```python
from build123d import *

# Parameters (mm, degrees)
BOSS_EXTRUDE1_DEPTH  = 10.16
SKETCH3_R            = 1.27
CUT_EXTRUDE1_DEPTH   = 10.16
SKETCH4_W            = 8.255
SKETCH4_H            = 7.62
CUT_EXTRUDE2_DEPTH   = 10.16
FILLET2_R            = 0.508
FILLET3_R            = 1.27
SKETCH6_W            = 84.495652993
SKETCH6_H            = 50.182540269
CUT_EXTRUDE3_DEPTH   = 27.94
CUT_EXTRUDE4_DEPTH   = 27.94
CUT_EXTRUDE5_DEPTH   = 40.132
FILLET4_R            = 2.54
FILLET2_OF_MIRROR1_R = 0.508
FILLET3_OF_MIRROR1_R = 1.27
FILLET4_OF_MIRROR1_R = 2.54


with BuildPart() as part:
    # Sketch1 → Boss-Extrude1 (new body)
    with BuildSketch(Plane(origin=(0, 0, 0), x_dir=(1, 0, 0), z_dir=(0, 1, 0))):
        with BuildLine():
            Line((-58.188733064, -33.517116066), (5.311266936, -33.517116066))
            Line((5.311266936, -33.517116066), (5.311266936, 14.742883934))
            Line((5.311266936, 14.742883934), (-53.108733064, 14.742883934))
            ThreePointArc((-53.108733064, 14.742883934), (-56.700835512, 13.254986382), (-58.188733064, 9.662883934))
            Line((-58.188733064, 9.662883934), (-58.188733064, -0.370116066))
            Line((-58.188733064, -0.370116066), (-66.443733064, -0.370116066))
            Line((-66.443733064, -0.370116066), (-66.443733064, -5.450116066))
            Line((-66.443733064, -5.450116066), (-58.188733064, -5.450116066))
            Line((-58.188733064, -5.450116066), (-58.188733064, -33.517116066))
        make_face()
    boss_extrude1 = extrude(amount=BOSS_EXTRUDE1_DEPTH)

    # Sketch3 → Cut-Extrude1 (cut)
    with BuildSketch(Plane(origin=(0, 10.16, 0), x_dir=(1, 0, 0), z_dir=(0, 1, 0))):
        with Locations(Location((-63.903733064, -2.910116066, 0), (0, 0, 270))):
            Circle(SKETCH3_R)
    cut_extrude1 = extrude(amount=-CUT_EXTRUDE1_DEPTH, mode=Mode.SUBTRACT)

    # Sketch4 → Cut-Extrude2 (cut)
    with BuildSketch(Plane.XY.offset(5.450116066)):
        with Locations((-62.316233064, 6.35)):
            Rectangle(SKETCH4_W, SKETCH4_H)
    cut_extrude2 = extrude(amount=-CUT_EXTRUDE2_DEPTH, mode=Mode.SUBTRACT)

    # Fillet2
    fillet2_edges = [part.edges().sort_by_distance(p)[0] for p in [
        (-58.188733064, 1.27, 5.450116066),
        (-58.188733064, 1.27, 0.370116066),
        (-58.188733064, 2.54, 2.910116066),
    ]]
    fillet(fillet2_edges, radius=FILLET2_R)

    # Fillet3
    fillet3_edges = [part.edges().sort_by_distance(p)[0] for p in [
        (-66.443733064, 1.27, 5.450116066),
        (-66.443733064, 1.27, 0.370116066),
    ]]
    fillet(fillet3_edges, radius=FILLET3_R)

    # Sketch6 → Cut-Extrude3 (cut)
    with BuildSketch(Plane(origin=(5.311266936, 0, 0), x_dir=(0, 0, -1), z_dir=(1, 0, 0))):
        with Locations((-10.301713583, -2.397336113)):
            Rectangle(SKETCH6_W, SKETCH6_H)
    cut_extrude3 = extrude(amount=-CUT_EXTRUDE3_DEPTH, mode=Mode.SUBTRACT)

    # Sketch7 → Cut-Extrude4 (cut)
    with BuildSketch(Plane(origin=(0, 10.16, 0), x_dir=(1, 0, 0), z_dir=(0, 1, 0))):
        with BuildLine():
            Line((-22.628733064, 14.742883934), (-27.708733064, 14.742883934))
            ThreePointArc((-27.708733064, 14.742883934), (-24.116630616, 13.254986382), (-22.628733064, 9.662883934))
            Line((-22.628733064, 9.662883934), (-22.628733064, 14.742883934))
        make_face()
    cut_extrude4 = extrude(amount=-CUT_EXTRUDE4_DEPTH, mode=Mode.SUBTRACT)

    # Sketch8 → Cut-Extrude5 (cut)
    with BuildSketch(Plane.ZY.offset(58.188733064)):
        with BuildLine():
            Line((33.517116066, 10.16), (33.517116066, 8.89))
            Line((33.517116066, 8.89), (33.517116066, 7.62))
            ThreePointArc((33.517116066, 7.62), (32.619090454, 7.991974388), (32.247116066, 8.89))
            Line((32.247116066, 8.89), (32.247116066, 10.16))
            Line((32.247116066, 10.16), (33.517116066, 10.16))
        make_face()
    cut_extrude5 = extrude(amount=-CUT_EXTRUDE5_DEPTH, mode=Mode.SUBTRACT)

    # Fillet4
    fillet4_edges = [part.edges().sort_by_distance(p)[0] for p in [
        (-24.116630616, 10.16, -13.254986382),
        (-22.628733064, 10.16, 11.292116066),
        (-40.408733064, 10.16, -14.742883934),
        (-56.700835512, 10.16, -13.254986382),
        (-58.188733064, 10.16, 11.292116066),
    ]]
    fillet(fillet4_edges, radius=FILLET4_R)


with BuildPart() as mirror1_1:
    # Mirror1: Boss-Extrude1 across plane
    add(boss_extrude1.mirror(Plane(origin=(-58.188733064, 10.16, 33.517116066), x_dir=(1, 0, 0), z_dir=(0, 0, -1))))

    # Mirror1 2: Cut-Extrude1, Cut-Extrude2, Cut-Extrude3, Cut-Extrude4, Cut-Extrude5 across plane
    add(cut_extrude1.mirror(Plane(origin=(-58.188733064, 10.16, 33.517116066), x_dir=(1, 0, 0), z_dir=(0, 0, -1))), mode=Mode.SUBTRACT)
    add(cut_extrude2.mirror(Plane(origin=(-58.188733064, 10.16, 33.517116066), x_dir=(1, 0, 0), z_dir=(0, 0, -1))), mode=Mode.SUBTRACT)
    add(cut_extrude3.mirror(Plane(origin=(-58.188733064, 10.16, 33.517116066), x_dir=(1, 0, 0), z_dir=(0, 0, -1))), mode=Mode.SUBTRACT)
    add(cut_extrude4.mirror(Plane(origin=(-58.188733064, 10.16, 33.517116066), x_dir=(1, 0, 0), z_dir=(0, 0, -1))), mode=Mode.SUBTRACT)
    add(cut_extrude5.mirror(Plane(origin=(-58.188733064, 10.16, 33.517116066), x_dir=(1, 0, 0), z_dir=(0, 0, -1))), mode=Mode.SUBTRACT)

    # Fillet2 of Mirror1
    fillet2_of_mirror1_edges = [mirror1_1.edges().sort_by_distance(p)[0] for p in [
        (-58.188733064, 1.27, 61.584116066),
        (-58.188733064, 1.27, 66.664116066),
        (-58.188733064, 2.54, 64.124116066),
    ]]
    fillet(fillet2_of_mirror1_edges, radius=FILLET2_OF_MIRROR1_R)

    # Fillet3 of Mirror1
    fillet3_of_mirror1_edges = [mirror1_1.edges().sort_by_distance(p)[0] for p in [
        (-66.443733064, 1.27, 61.584116066),
        (-66.443733064, 1.27, 66.664116066),
    ]]
    fillet(fillet3_of_mirror1_edges, radius=FILLET3_OF_MIRROR1_R)

    # Fillet4 of Mirror1
    fillet4_of_mirror1_edges = [mirror1_1.edges().sort_by_distance(p)[0] for p in [
        (-24.116630616, 10.16, 80.289218515),
        (-22.628733064, 10.16, 55.742116066),
        (-40.408733064, 10.16, 81.777116066),
        (-56.700835512, 10.16, 80.289218515),
        (-58.188733064, 10.16, 55.742116066),
    ]]
    fillet(fillet4_of_mirror1_edges, radius=FILLET4_OF_MIRROR1_R)


with BuildPart() as part_1:
    add(part.part)

    # Mirror1 united with what the copies touc: union Mirror1_1
    add(mirror1_1.part)


solid = part_1.part
```
Geometry: final body of the model. Coordinates: model frame, mm. A direction names the side the tool comes from. Round coordinates to 2 decimals unless told otherwise and drop trailing zeros. Order: outer loops, then holes, each group sorted by start corner. A loop starts at its lowest first (then second) coordinate and runs counter-clockwise, first axis right, second up. Notation, with made-up numbers: (-21, -20.5) - (30, -20.5) arc R27 cw to (30, 9.5) - close; hole circle Ø1 at (-16.75, 78). An arc over 180 degrees is marked (long way). Use CSV: the item, a comma, the result in double quotes. Start each with the question number.
Q1. Section query C-C (z = 18.5). Return loops of the section in (x, y), and give its area (3 significant figures).
Q2. Access query for faces 1 (the face through (-58.189, 4, 34)), 2 (the face through (-62, 2.54, 3)), 3 (the face through (-65.144, 1.288, 2.635)). Directions: +Z, -Z, +X, -X, +Y, -Y. A direction counts if a zero-diameter tool reaches every point of the face in a straight line with its end or side. Return the directions, or none.
Q3. Mould query, pull axis Z, two halves, no side actions, for faces 4 (the face through (-62, 1, 66.664)), 5 (the face through (-64.39, 1.29, 62.95)), 6 (the face through (-40, 4, -14.743)), 7 (the face through (-62, 2.54, 64)). Classes: +Z half, -Z half, draft (parallel to the pull), parting line (faces both ways), or undercut.
Q4. Section query B-B (y = 4.5). Return loops of the section in (x, z).
Q5. Section query A-A (x = -61). Return loops of the section in (y, z).
Q6. Material intervals for line 1 along X through (y, z) = (1, 17); line 2 along Z through (x, y) = (-52.5, 9.75); line 3 along Z through (x, y) = (-25.5, 8.5), sorted ascending. Write a range as from..to.
Q7. First-contact query: pin 1 (1.5 mm diameter, centred on y = 6.5, z = 64.5, fed in from -X); pin 2 (1.3 mm diameter, centred on x = -61, y = 1.5, fed in from -Z); pin 3 (1.4 mm diameter, centred on x = -41, y = 10, fed in from +Z); pin 4 (1 mm diameter, centred on x = -58.5, z = 21.5, fed in from -Y). Flat tips, straight axial feed; report the tip coordinate or a pass-through.
Result set:
1,outline,"(-58.19, 0) - (-22.63, 0) - (-22.63, 7.62) arc R2.54 ccw to (-25.17, 10.16) - (-55.65, 10.16) arc R2.54 ccw to (-58.19, 7.62) - close"
1,area,"359 mm2"
2,face 1,"-X, +Y"
2,face 2,"+Z, -Z, -X, +Y"
2,face 3,"+Y, -Y"
3,face 4,"+Z half"
3,face 5,"undercut"
3,face 6,"-Z half"
3,face 7,"draft"
4,outline,"(-58.19, -9.66) arc R5.08 ccw to (-53.11, -14.74) - (-27.71, -14.74) arc R5.08 ccw to (-22.63, -9.66) - (-22.63, 76.7) arc R5.08 ccw to (-27.71, 81.78) - (-53.11, 81.78) arc R5.08 ccw to (-58.19, 76.7) - close"
5,outline,"(0, 0.37) - (2.54, 0.37) - (2.54, 5.45) - (0, 5.45) - close; (0, 61.58) - (2.54, 61.58) - (2.54, 66.66) - (0, 66.66) - close"
6,line 1,"x = -58.19..-22.63"
6,line 2,"z = -13.59..32.25, 34.79..80.62"
6,line 3,"z = -14.06..32.31, 34.73..81.1"
7,pin 1,"stops at x = -58.19"
7,pin 2,"stops at z = 0.37"
7,pin 3,"stops at z = 81.14"
7,pin 4,"stops at y = 0"
